Can you work these out from the drawing? Everything is in mm from the part's minimum corner. A direction names the side the tool comes from. Coordinates: 2 decimals unless noted, no trailing zeros. Order: outer loops, then holes, each group sorted by start corner. A loop starts at its lowest first (then second) coordinate and runs counter-clockwise, first axis right, second up. Notation, with made-up numbers: (-2.5, 87.25) - (44.5, 87.25) arc R14 cw to (44.5, 108.25) - close; hole circle Ø9 at (61.25, 27.25). An arc over 180 degrees is marked (long way). Use a Markdown table: item, result. Add a question column.
(1) On a 3-axis mill with a long thin cutter (end or side, diameter ignored), from which of +Z, -Z, +X, -X, +Y, -Y can I reach the whole of each face in a straight line? I mean the marked faces 1, 2 and 3. Say none if no direction works.
(2) We'd pull the mould along Z, two halves only. Please class the marked faces 4, 5 and 6: pulls with the +Z half, pulls with the -Z half, needs draft (parallel to the pull), parting line crosses it, or undercut.
(3) If I drill on L1, parallel to X at y = 2.5, z = 9.75; L2, parallel to X at y = 1.75, z = 10.5; L3, parallel to Z at x = 2, y = 5, over which ranges is the centre line in solid material (lowest first)? Write a range as [from, to].
(4) I want a section at B-B (y = 1.5). List the corners of the cut face in (x, z) for me.
(5) I want a section at C-C (z = 9.75). List the corners of the cut face in (x, y) for me.
(6) For pin 1 Ø2 at (x, z) = (1.5, 14) entering from -Y; pin 2 Ø4.5 at (x, z) = (18.5, 14.5) entering from +Y; pin 3 Ø1.5 at (x, z) = (15, 9.75) entering from -Y, each with a flat end and sliding along its axis, tell me the tip position at first contact or that it passes through.
(7) I want a section at D-D (x = 11.75). List the corners of the cut face in (y, z) for me, and give its area (3 significant figures).
(8) I want a section at A-A (x = 15). List the corners of the cut face in (y, z) for me.
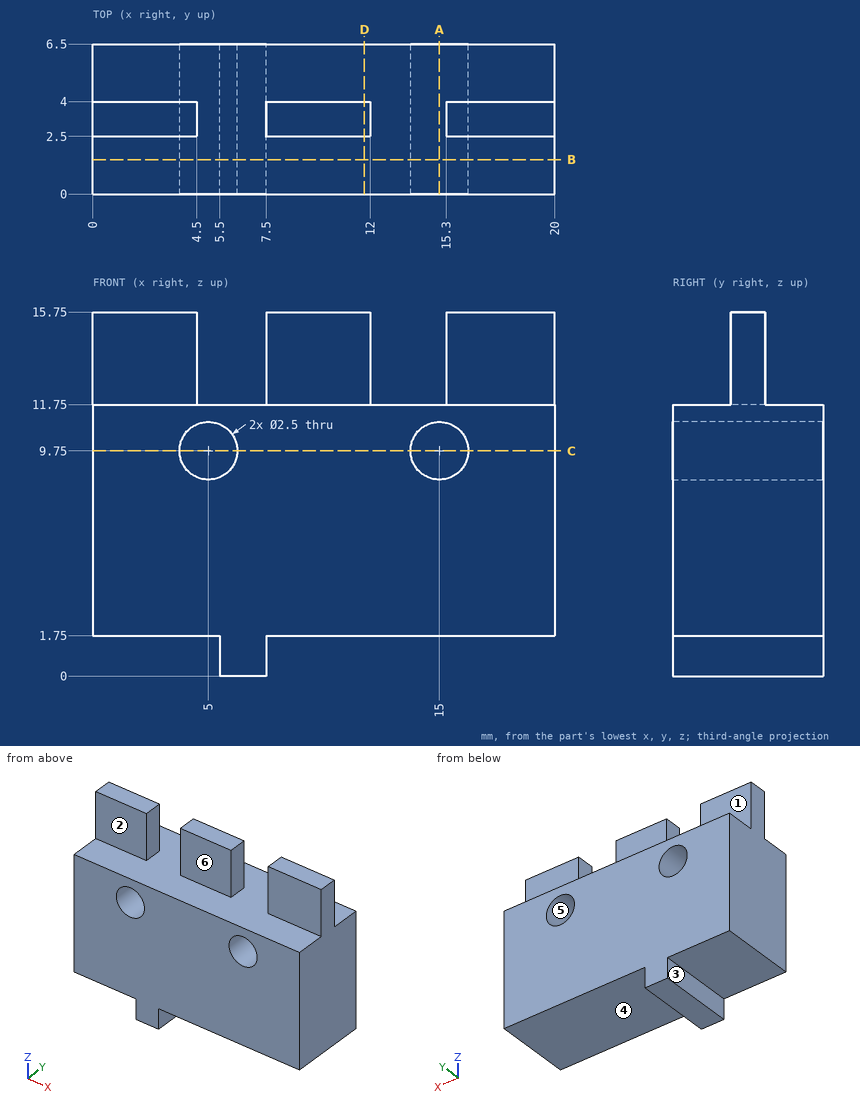
Answers follow:
| question | item | result |
|---|---|---|
| 1 | face 1 | +Z, +X, -X, +Y |
| 1 | face 2 | +Z, +X, -X, -Y |
| 1 | face 3 | -Z, -X, +Y, -Y |
| 2 | face 4 | pulls with the -Z half |
| 2 | face 5 | undercut |
| 2 | face 6 | needs draft |
| 3 | L1 | x = [0, 3.75], [6.25, 13.75], [16.25, 20] |
| 3 | L2 | x = [0, 4], [6, 14], [16, 20] |
| 3 | L3 | z = [1.75, 11.75] |
| 4 | outline | (0, 1.75) - (5.5, 1.75) - (5.5, 0) - (7.5, 0) - (7.5, 1.75) - (20, 1.75) - (20, 11.75) - (0, 11.75) - close; hole circle Ø2.5 at (5, 9.75); hole circle Ø2.5 at (15, 9.75) |
| 5 | outline | (0, 0) - (3.75, 0) - (3.75, 6.5) - (0, 6.5) - close; (6.25, 0) - (13.75, 0) - (13.75, 6.5) - (6.25, 6.5) - close; (16.25, 0) - (20, 0) - (20, 6.5) - (16.25, 6.5) - close |
| 6 | pin 1 | stops at y = 2.5 |
| 6 | pin 2 | stops at y = 4 |
| 6 | pin 3 | passes through |
| 7 | outline | (0, 1.75) - (6.5, 1.75) - (6.5, 11.75) - (4, 11.75) - (4, 15.75) - (2.5, 15.75) - (2.5, 11.75) - (0, 11.75) - close |
| 7 | area | 71.0 mm² |
| 8 | outline | (0, 1.75) - (6.5, 1.75) - (6.5, 8.5) - (0, 8.5) - close; (0, 11) - (6.5, 11) - (6.5, 11.75) - (0, 11.75) - close |
